Read the model definition and answer for the solid it produces. Units are mm, in the model's axes. Face numbers are marked on the shaded views. A direction names the side the tool comes from. Coordinates: 2 decimals unless noted, no trailing zeros. Order: outer loops, then holes, each group sorted by start corner. A loop starts at its lowest first (then second) coordinate and runs counter-clockwise, first axis right, second up. Notation, with made-up numbers: M -22.5,-15.5 L 25.5,-15.5 A18 cw 25.5,-9.5 Z; hole C 21,70 d6. An arc over 180 degrees is marked long. One line per question, with ' | ' between items. Start each with the question number.
1) Find section A-A, the plane x = -6.35. Write down the section's boundary in (y, z) (3 decimals).
2) Consider probe 1 along Y at (x, z) = (-31.75, 17.25); probe 2 along Y at (x, z) = (-6, 33); probe 3 along Z at (x, y) = (49, 14) (3 decimals). Determine where each line is inside the solid, lowest interval first.
3) Given P1, Ø5, axis at x = -6.35, y = 9.525, coming from the -Z side (3 decimals); P2, Ø7.5, axis at x = 101.6, y = 0, coming from the -Z side; P3, Ø2, axis at y = 11.5, z = 26, coming from the +X side; P4, Ø2, axis at y = -12, z = 45.5, coming from the -X side, each flat-ended and moving along its own axis, determine where each tip first touches the part or whether it passes through.
4) Find section D-D, the plane x = 101.6. Write down the section's boundary in (y, z) (3 decimals), plus the area to 3 significant figures.
5) A tool of negligible diameter and unlimited length cuts with its end or side. For the marked faces 1, 2 and 3, from which of +Z, -Z, +X, -X, +Y, -Y can it reach the whole face along a straight path? Write none if from no direction.
6) Find section B-B, the plane z = 45. Write down the section's boundary in (x, y) (3 decimals).
7) Find section C-C, the plane y = 16. Write down the section's boundary in (x, z) (3 decimals), plus the area to 3 significant figures.
from build123d import *

# Parameters (mm, degrees)
BOSS_EXTRUDE1_DEPTH = 3.175
SKETCH2_W           = 12.7
SKETCH2_H           = 50.8
BOSS_EXTRUDE2_DEPTH = 31.75
FILLET1_R           = 12.7
BOSS_EXTRUDE3_DEPTH = 3.175
FILLET2_R           = 38.1
SKETCH4_R           = 2.15265
CUT_EXTRUDE1_DEPTH  = 38.1
FILLET3_R           = 25.4
CUT_EXTRUDE4_REACH  = 131.047
SKETCH7_R           = 3.175


# Some blends are built 0.0001 mm under size
with BuildPart() as part:
    # Sketch1 → Boss-Extrude1 (new body)
    with BuildSketch(Plane.XY.offset(15.875)):
        Polygon((-38.1, 25.4), (-38.1, -25.4), (-25.4, -25.4), (0, -25.4), (0, 25.4), align=None)
    extrude(amount=BOSS_EXTRUDE1_DEPTH)

    # Sketch2 → Boss-Extrude2 (add)
    with BuildSketch(Plane.XY.offset(50.8)):
        with Locations((-6.35, 0)):
            Rectangle(SKETCH2_W, SKETCH2_H)
    extrude(amount=-BOSS_EXTRUDE2_DEPTH)

    # Fillet1
    fillet1_edges = [part.edges().sort_by_distance(p)[0] for p in [
        (-12.7, 0, 19.05),
    ]]
    fillet(fillet1_edges, radius=FILLET1_R)

    # Sketch3 → Boss-Extrude3 (add)
    with BuildSketch(Plane.XY.offset(50.8)):
        Polygon((0, 25.4), (101.6, 25.4), (120.65, 25.4), (120.65, -25.4), (0, -25.4), (-12.7, -25.4), (-12.7, 25.4), align=None)
    extrude(amount=BOSS_EXTRUDE3_DEPTH)

    # Fillet2
    # the kernel refuses this fillet: 38.1 mm, written as the material it adds along each edge
    with BuildSketch(Plane(origin=(0, -25.4, 50.8), x_dir=(0, 0, -1), z_dir=(0, 1, 0))) as fillet2_piece_1:
        with BuildLine():
            CenterArc((38.1, -37.967477859), FILLET2_R, 94.780191847, 85.219808153)
            Line((0, -37.967477859), (-0.762, -37.967477859))
            Line((-0.762, -37.967477859), (-0.762, 0))
            Line((-0.762, 0), (0, 0.762))
            ThreePointArc((0, 0.762), (17.4625, 0.762), (34.8615, 0.759349557))
            Line((34.8615, 0.759349557), (34.925, 0))
        make_face()
    extrude(amount=50.8)

    # Sketch4 → Cut-Extrude1 (cut)
    with BuildSketch(Plane.XY.offset(53.975)):
        with Locations((-6.35, 9.525)):
            Circle(SKETCH4_R)
        with Locations((-31.75, 9.525)):
            Circle(SKETCH4_R)
        with Locations((-6.35, -9.525)):
            Circle(SKETCH4_R)
        with Locations((-31.75, -9.525)):
            Circle(SKETCH4_R)
    extrude(amount=-CUT_EXTRUDE1_DEPTH, mode=Mode.SUBTRACT)

    # Fillet3
    fillet3_edges = [part.edges().sort_by_distance(p)[0] for p in [
        (120.65, -25.4, 52.3875),
        (120.65, 25.4, 52.3875),
    ]]
    fillet(fillet3_edges, radius=FILLET3_R - 0.0001)  # a hair under: the kernel refuses the full size

    # Sketch7 → Cut-Extrude4 (cut, up to next)
    with BuildSketch(Plane.XY.offset(53.975), mode=Mode.PRIVATE) as cut_extrude4_sk1:
        with Locations((101.6, 0)):
            Circle(SKETCH7_R)
    cut_extrude4_tool1 = extrude(cut_extrude4_sk1.sketch, amount=-CUT_EXTRUDE4_REACH, mode=Mode.PRIVATE) & part.part
    add(cut_extrude4_tool1.solids().sort_by_distance((101.6, 0, 53.975))[0], mode=Mode.SUBTRACT)


solid = part.part
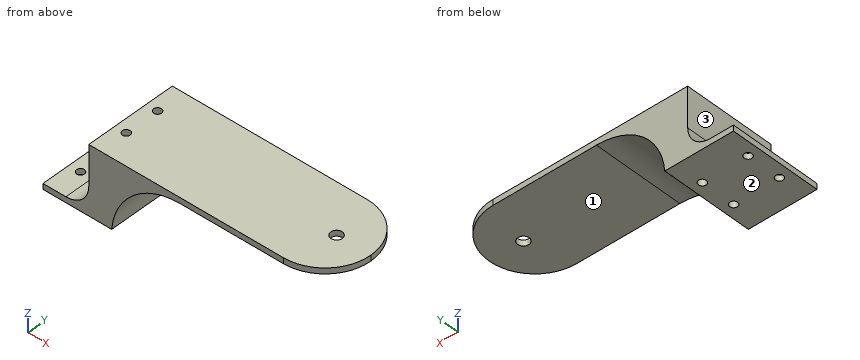
Report:
1) outline: M -25.4,15.875 L -11.678,15.875 L -11.678,53.975 L -25.4,53.975 Z; M -7.372,15.875 L 7.372,15.875 L 7.372,53.975 L -7.372,53.975 Z; M 11.678,15.875 L 25.4,15.875 L 25.4,53.975 L 11.678,53.975 Z
2) probe 1: y = -25.4 to -11.68, -7.37 to 7.37, 11.68 to 25.4 | probe 2: y = -25.4 to -11.65, -7.4 to 7.4, 11.65 to 25.4 | probe 3: z = 50.8 to 53.975
3) P1: stops at z = 15.875 | P2: stops at z = 50.8 | P3: stops at x = 2.65 | P4: stops at x = -12.7
4) outline: M -24.593,50.8 L -3.175,50.8 L -3.175,53.975 L -24.593,53.975 Z; M 3.175,50.8 L 24.593,50.8 L 24.593,53.975 L 3.175,53.975 Z | area: 136 mm^2
5) face 1: -Z, +X, +Y, -Y | face 2: -Z, +X, -X, +Y, -Y | face 3: +Z, -X, +Y, -Y
6) outline: M -12.7,-25.4 L 17.761,-25.4 L 17.761,25.4 L -12.7,25.4 Z; hole C -6.35,-9.525 d4.305; hole C -6.35,9.525 d4.305
7) outline: M -38.1,15.875 L 0,15.875 A38.1 cw 37.967,50.8 L 114.977,50.8 L 114.977,53.975 L -12.7,53.975 L -12.7,31.75 A12.7 cw -25.4,19.05 L -38.1,19.05 Z | area: 1,270 mm^2
